```python
from build123d import *

# Parameters (mm, degrees)
SKETCH1_W                      = 20.32
SKETCH1_H                      = 9.525
EXTRUDE1_DEPTH                 = 7.62
F_3_16_0_1875_DIAMETER_HOLE1_D = 4.7625
SKETCH4_W                      = 11.43
SKETCH4_H                      = 9.525
EXTRUDE2_DEPTH                 = 4.191
CHAMFER1_SIZE                  = 1.905


with BuildPart() as part:
    # Sketch1 → Extrude1 (new body)
    with BuildSketch(Plane.XY):
        with Locations((10.16, 4.7625)):
            Rectangle(SKETCH1_W, SKETCH1_H)
    extrude(amount=EXTRUDE1_DEPTH)

    # 3/16 (0.1875) Diameter Hole1 (through all)
    with Locations(Plane(origin=(4.042308369, -0.495150795, 7.62), x_dir=(-1, 0, 0), z_dir=(0, 0, 1))):
        with Locations((-9.927691631, -5.257650795)):
            Hole(F_3_16_0_1875_DIAMETER_HOLE1_D / 2)

    # Sketch4 → Extrude2 (cut)
    with BuildSketch(Plane.XY.offset(7.62)):
        with Locations((14.605, 4.7625)):
            Rectangle(SKETCH4_W, SKETCH4_H)
    extrude(amount=-EXTRUDE2_DEPTH, mode=Mode.SUBTRACT)

    # Chamfer1
    chamfer1_edges = [part.edges().sort_by_distance(p)[0] for p in [
        (20.32, 9.525, 1.7145),
        (20.32, 0, 1.7145),
        (8.89, 9.525, 5.5245),
        (8.89, 0, 5.5245),
        (0, 9.525, 3.81),
        (0, 0, 3.81),
    ]]
    chamfer(chamfer1_edges, length=CHAMFER1_SIZE)

    # Sketch5 → CBORE for #4 Socket Head Cap Screw1 (revolve, cut)
    with BuildSketch(Plane(origin=(3.81, 4.7625, 0), x_dir=(0, 1, 0), z_dir=(1, 0, 0))):
        Polygon((0, 0), (0, 7.62), (1.905, 7.62), (1.5875, 7.3025), (1.5875, 1.524), (1.6002, 1.524), (1.6002, 0.3048), (1.905, 0), align=None)
    revolve(axis=Axis((3.81, 4.7625, -6.35), (0, 0, 1)), mode=Mode.SUBTRACT)


solid = part.part
```
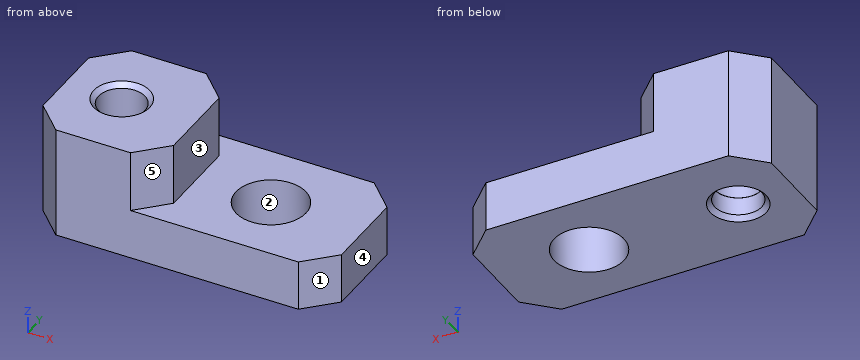
For this review, take the finished solid that the model builds, in its own axes (mm). Face numbers are marked on the shaded views. A direction names the side the tool comes from. Coordinates: 2 decimals unless noted, no trailing zeros. Loops run counter-clockwise (first coordinate to the right, second up) from the corner with the lowest first, then second, coordinate; pieces in that order, holes last. Notation, with made-up numbers: (8.25, -2) -> (25.25, -2) arc R31 ccw to (25.25, 36) -> close; hole circle Ø6 at (56.25, 33). An arc over 180 degrees is marked (long way). Return JSON: item names as keys, results as strings. Group by question number.
(1) Consider section C-C, the plane z = 3. Count the separate pieces of the cut face and the enclosed holes in it, plus the area to 3 significant figures.
(2) To check wall thickness, follow L1, parallel to Y at x = 3.81, z = 1 (3 decimals); L2, parallel to Z at x = 17, y = 2.5; L3, parallel to X at y = 6.75, z = 5.75. State the ranges of each line that lie inside material, in increasing order.
(3) Mouldability with a two-part tool opening along Y and no side actions: class the marked faces 1, 2 and 3 as pulls with the +Y half, pulls with the -Y half, needs draft (parallel to the pull), parting line crosses it, or undercut.
(4) For pin 1 Ø5 at (x, y) = (16, 7) entering from +Z; pin 2 Ø4 at (x, y) = (17, 2) entering from -Z; pin 3 Ø2 at (y, z) = (4, 6) entering from +X; pin 4 Ø3.5 at (x, y) = (3.81, 4.76) entering from -Z, all flat-tipped, find the tip position at first contact; note any pin that passes through.
(5) Tool access review of the marked faces 4 and 5: name each direction out of +Z, -Z, +X, -X, +Y, -Y from which nothing blocks a thin tool from reaching the whole face with its end or side.
(6) Consider section A-A, the plane x = 13.97. Give the boundary of the cut face in (y, z) (3 decimals).
Results below:
{
 "1": {"separate pieces": "1", "enclosed holes": "2", "area": "161 mm2"},
 "2": {"L1": "y = 0 to 3.162, 6.363 to 9.525", "L2": "z = 0 to 3.43", "L3": "x = 0 to 8.89"},
 "3": {"face 1": "pulls with the -Y half", "face 2": "undercut", "face 3": "needs draft"},
 "4": {"pin 1": "stops at z = 3.43", "pin 2": "stops at z = 0", "pin 3": "stops at x = 8.89", "pin 4": "stops at z = 0.15"},
 "5": {"face 4": "+Z, -Z, +X, +Y, -Y", "face 5": "+Z, +X, -Y"},
 "6": {"outline": "(0, 0) -> (2.381, 0) -> (2.381, 3.429) -> (0, 3.429) -> close; (7.144, 0) -> (9.525, 0) -> (9.525, 3.429) -> (7.144, 3.429) -> close"}
}
